Check sheet for the modelled part. Datum: model origin and axes. Units: mm. A direction names the side the tool comes from. Round coordinates to 2 decimals unless told otherwise and drop trailing zeros. Order: outer loops, then holes, each group sorted by start corner. A loop starts at its lowest first (then second) coordinate and runs counter-clockwise, first axis right, second up.
(1) Tool access check on faces 5 (the flat face through (-12.2, -10.9, -5.2)), 6 (the flat face through (-24, -9.655, 0)), 7 (the flat face through (0.87, 11.14, -3.789)), 8 (the cylindrical face through (11.95, -4, 4.35)). Record the directions out of +Z, -Z, +X, -X, +Y, -Y that give a thin tool (end or side, any length) a straight path to the whole face; none if there is none.
(2) Sectioned sample at B-B, the plane x = -21. Enter the section's corners in (y, z) (3 decimals).
(3) Thickness scan on probe 1 along Y at (x, z) = (0, 4.35) (3 decimals); probe 2 along Y at (x, z) = (0, -3.7) (3 decimals); probe 3 along X at (y, z) = (-2.75, 5). Record the ranges inside material, lowest first.
(4) Sectioned sample at A-A, the plane z = 0. Enter the section's corners in (x, y) (3 decimals).
(5) Depth check by flat-ended pin: pin 1 (1.8 mm diameter, centred on x = 5, y = -13.5, fed in from +Z); pin 2 (5.5 mm diameter, centred on x = -19, y = -12, fed in from +Z) (3 decimals); pin 3 (15.5 mm diameter, centred on x = 6, y = 4.5, fed in from -Z). Enter the tip coordinate at first touch or a pass-through.
(6) Mould release check, pull along X, two halves, no side actions. Record for faces 1 (the flat face through (2, 10, -3.5)), 2 (the flat face through (13.907, -4.335, -5.725)), 3 (the flat face through (27.135, -12.271, 5.342)), 4 (the flat face through (-15.11, -3.27, 0.09)): released by +X, released by -X, zero draft, split by the parting line, or undercut.
```python
from build123d import *

# Parameters (mm, degrees)
BOSS_EXTRUDE1_DEPTH     = 6.575
SKETCH8_R               = 2.400000000000001
CUT_EXTRUDE3_DEPTH      = 39.155592587632775
CHAMFER1_SIZE           = 2.5
BOSS_EXTRUDE2_DEPTH     = 1.71
FILLET1_R               = 2
CUT_EXTRUDE4_DEPTH      = 1.725
CUT_EXTRUDE5_START      = -13.15
CUT_EXTRUDE5_DEPTH      = 1.725
CUT_EXTRUDE_THIN5_START = 7
CUT_EXTRUDE_THIN5_DEPTH = 26.81086056039093
CUT_EXTRUDE_THIN6_START = -7
CUT_EXTRUDE_THIN6_DEPTH = 26.81086056039093
FILLET2_R               = 2


# Read off the part's stored shape, not the designer's step: Cut-Extrude5
with BuildPart() as part:
    # Sketch1 → Revolve1 (revolve)
    with BuildSketch(Plane(origin=(0, 0, 0), x_dir=(0, 0, -1), z_dir=(1, 0, 0)), mode=Mode.PRIVATE) as revolve1_sk:
        Polygon((-7.0985121547008365, 5.999999999999999), (-3.4357973085956934, 6), (1.3e-15, 6), (3.4357973085956957, 6), (3.499999999999999, 6), (3.499999999999999, 4), (-7.0985121547008365, 3.999999999999999), align=None)
        Polygon((3.4357973085956957, 6), (1.3e-15, 6), (-3.4357973085956934, 6), (-3.4357973085956934, 9.999999999999998), (3.435797308595695, 9.999999999999998), align=None)
        Polygon((3.5000000000000013, 9.999999999999998), (3.435797308595695, 9.999999999999998), (-3.4357973085956934, 9.999999999999998), (-3.4999999999999996, 9.999999999999998), (-3.5000000000000018, 11), (-1.18e-15, 11), (3.499999999999999, 11), align=None)
        Polygon((3.789167362820558, 11), (3.499999999999999, 11), (-1.18e-15, 11), (-3.5000000000000018, 11), (-3.789167362820557, 11), (-3.789167362820557, 12.6), (5.8e-16, 12.6), (3.789167362820558, 12.6), align=None)
        Polygon((4.8500000000000005, 12.6), (3.789167362820558, 12.6), (5.8e-16, 12.6), (-3.789167362820557, 12.6), (-4.849999999999999, 12.6), (-4.849999999999999, 14.815), (0, 14.815), (4.8500000000000005, 14.815), align=None)
    revolve(revolve1_sk.sketch.rotate(Axis((0, 0, 11.627586075142245), (0, 0, -1)), 90), axis=Axis((0, 0, 11.627586075142245), (0, 0, -1)))

    # Sketch2 → Boss-Extrude1 (add, symmetric)
    with BuildSketch(Plane.XY):
        Polygon((28.402103283084184, -9.655000000000001), (15.601451795624948, -9.655000000000001), (12.102278163852397, -9.655000000000001), (12.500000000000004, -14.815000000000001), (28.402103283084184, -14.815), align=None)
        with BuildLine():
            ThreePointArc((14.771362958963898, 1.1362487995810626), (10.066049350023114, 10.87009086819882), (-3.5216e-13, 14.815000000000007))
            Line((0, 14.815000000000005), (0, 12.6))
            ThreePointArc((3.5261e-13, 12.600000000000001), (10.420944759538665, 7.082648538410167), (11.71553796349213, -4.6374745525959185))
            Line((11.71553796349213, -4.6374745525959185), (12.10227816385239, -9.655000000000001))
            Line((12.102278163852397, -9.655000000000001), (15.601451795624948, -9.655000000000001))
            Line((15.601451795624948, -9.655000000000001), (14.7713629589639, 1.1362487995810628))
        make_face()
        with BuildLine():
            Line((0, 12.6), (0, 14.815000000000005))
            ThreePointArc((-3.5216e-13, 14.815000000000007), (-10.066049350023373, 10.87009086819858), (-14.771362958963902, 1.136248799581064))
            Line((-14.7713629589639, 1.1362487995810628), (-15.601451795624941, -9.655000000000005))
            Line((-15.601451795624941, -9.655000000000005), (-12.10227816385239, -9.655000000000005))
            Line((-12.102278163852386, -9.655000000000005), (-11.71553796349213, -4.6374745525959185))
            ThreePointArc((-11.71553796349213, -4.637474552595917), (-10.420944759538465, 7.08264853841046), (3.5261e-13, 12.600000000000001))
        make_face()
        Polygon((-12.10227816385239, -9.655000000000005), (-15.601451795624941, -9.655000000000005), (-28.402103283084177, -9.655000000000006), (-28.402103283084177, -14.815000000000007), (-12.499999999999996, -14.815000000000005), align=None)
    extrude(amount=BOSS_EXTRUDE1_DEPTH, both=True)

    # Sketch8 → Cut-Extrude3 (cut, through all)
    with BuildSketch(Plane(origin=(0, -9.655000000000001, 0), x_dir=(1, 0, 0), z_dir=(0, 1, 0))):
        with Locations(Location((21.000000000000004, 0, 0), (0, 0, 270))):
            Circle(SKETCH8_R)
        with Locations(Location((-21.000000000000004, 0, 0), (0, 0, 90))):
            Circle(SKETCH8_R)
    extrude(amount=-CUT_EXTRUDE3_DEPTH, mode=Mode.SUBTRACT)

    # Chamfer1
    chamfer1_edges = [part.edges().sort_by_distance(p)[0] for p in [
        (-28.402103283084177, -12.235000000000007, -6.575),
        (28.402103283084184, -12.235, 6.575),
        (-28.402103283084177, -12.235000000000007, 6.575),
        (28.402103283084184, -12.235, -6.575),
    ]]
    chamfer(chamfer1_edges, length=CHAMFER1_SIZE)

    # Sketch9 → Boss-Extrude2 (add, symmetric)
    with BuildSketch(Plane.XY):
        with BuildLine():
            Line((-12.499999999999996, -14.815000000000007), (12.500000000000004, -14.815000000000001))
            Line((12.500000000000004, -14.815000000000001), (11.715537963492132, -4.637474552595919))
            ThreePointArc((11.715537963492132, -4.637474552595919), (-9.9e-16, -12.600000000000003), (-11.71553796349213, -4.6374745525959185))
            Line((-11.71553796349213, -4.6374745525959185), (-12.499999999999996, -14.815000000000007))
        make_face()
    extrude(amount=BOSS_EXTRUDE2_DEPTH, both=True)

    # Fillet1
    fillet1_edges = [part.edges().sort_by_distance(p)[0] for p in [
        (12.025078643317716, -8.653421786901651, -3.2800000000000002),
        (-12.025078643317713, -8.653421786901657, -3.2800000000000002),
        (-12.025078643317713, -8.653421786901657, 3.2799999999999994),
        (12.025078643317716, -8.653421786901651, 3.2799999999999994),
    ]]
    fillet(fillet1_edges, radius=FILLET1_R)

    # Sketch13 → Cut-Extrude4 (cut)
    with BuildSketch(Plane.XY.offset(6.575)):
        Polygon((-11.889993926761807, 0.705696375939659), (-17.610193659545324, 1.0452023711437894), (-14.425824047946865, 15.189187645015892), (3.1299229448728054, 17.38365601911835), (21.41715939572663, 11.678038246451958), (16.784392828177, 1.3884198701048673), (11.94080724759393, 0.7829716725319836), (0.5940928236877405, 11.678038246451958), align=None)
    extrude(amount=-CUT_EXTRUDE4_DEPTH, mode=Mode.SUBTRACT)

    # Cut-Extrude5 outline → Cut-Extrude5 (cut)
    with BuildSketch(Plane.XY.offset(6.575).offset(CUT_EXTRUDE5_START)):
        with BuildLine():
            Line((-14.791236442, 0.877891277), (-12.577865613, 0.746523021))
            ThreePointArc((-12.577865613, 0.746523021), (-0.057697816, 12.599867895), (12.57050125, 0.861683423))
            Line((12.57050125, 0.861683423), (14.771321629, 1.13678597))
            ThreePointArc((14.771321629, 1.13678597), (-0.000269379, 14.814999998), (-14.771362959, 1.1362488))
            Line((-14.771362959, 1.1362488), (-14.791236442, 0.877891277))
        make_face()
    extrude(amount=CUT_EXTRUDE5_DEPTH, mode=Mode.SUBTRACT)

    # Sketch14 → Cut-Extrude-Thin5 (cut, through all)
    with BuildSketch(Plane(origin=(0, 0, 0), x_dir=(0, 0, -1), z_dir=(1, 0, 0)).offset(CUT_EXTRUDE_THIN5_START)):
        Polygon((-4.849999999999999, 1.1367859701682461), (-6.575, -9.655000000000001), (-16.449646842920206, -8.076598996577228), (-14.724646842920205, 2.7151869735910195), align=None)
        Polygon((6.575, -9.655000000000001), (4.8500000000000005, 1.1367859701682461), (14.724646842920205, 2.7151869735910177), (16.449646842920206, -8.07659899657723), align=None)
    extrude(amount=CUT_EXTRUDE_THIN5_DEPTH, mode=Mode.SUBTRACT)

    # Sketch14<2> → Cut-Extrude-Thin6 (cut, through all)
    with BuildSketch(Plane(origin=(0, 0, 0), x_dir=(0, 0, -1), z_dir=(1, 0, 0)).offset(CUT_EXTRUDE_THIN6_START)):
        Polygon((-4.849999999999999, 1.1367859701682461), (-6.575, -9.655000000000001), (-16.449646842920206, -8.076598996577228), (-14.724646842920205, 2.7151869735910195), align=None)
        Polygon((6.575, -9.655000000000001), (4.8500000000000005, 1.1367859701682461), (14.724646842920205, 2.7151869735910177), (16.449646842920206, -8.07659899657723), align=None)
    extrude(amount=-CUT_EXTRUDE_THIN6_DEPTH, mode=Mode.SUBTRACT)

    # Fillet2
    fillet2_edges = [part.edges().sort_by_distance(p)[0] for p in [
        (15.601451795624948, -9.655000000000001, 0),
        (-15.601451795624941, -9.655000000000005, 0),
    ]]
    fillet(fillet2_edges, radius=FILLET2_R)


solid = part.part
```
Derived:
1. face 5: -Z, -Y
1. face 6: +Z, -Z, -X, +Y
1. face 7: -Z
1. face 8: +Z
2. outline: (-14.815, -6.575) - (-9.655, -6.575) - (-9.655, -2.4) - (-14.815, -2.4) - close; (-14.815, 2.4) - (-9.655, 2.4) - (-9.655, 6.575) - (-14.815, 6.575) - close
3. probe 1: y = -14.815 to -12.6, -6 to -4, 4 to 6, 12.6 to 14.815
3. probe 2: y = -14.815 to -11, 11 to 14.815
3. probe 3: x = -15.07 to -12.3, -5.33 to -2.9, 2.9 to 5.33, 12.3 to 15.07
4. outline: (-28.402, -14.815) - (-23.4, -14.815) - (-23.4, -9.655) - (-28.402, -9.655) - close; (-18.6, -14.815) - (18.6, -14.815) - (18.6, -9.655) - (17.454, -9.655) arc R2 cw to (15.459, -7.808) - (14.771, 1.136) arc R14.815 ccw to (-14.771, 1.136) - (-15.459, -7.808) arc R2 cw to (-17.454, -9.655) - (-18.6, -9.655) - close; (23.4, -14.815) - (28.402, -14.815) - (28.402, -9.655) - (23.4, -9.655) - close; hole circle Ø8 at (0, 0)
5. pin 1: stops at z = 4.85
5. pin 2: stops at z = 6.575
5. pin 3: stops at z = -4.96
6. face 1: undercut
6. face 2: zero draft
6. face 3: released by +X
6. face 4: released by -X
